Design review of the part built by this model. Coordinates are the model's own, in mm. Face numbers are marked on the shaded views. A direction names the side the tool comes from. Coordinates: 2 decimals unless noted, no trailing zeros. Loops run counter-clockwise (first coordinate to the right, second up) from the corner with the lowest first, then second, coordinate; pieces in that order, holes last. Notation, with made-up numbers: M 19.5,12.25 L 63.5,12.25 A6 cw 63.5,23.25 Z; hole C 50.5,-8.75 d2. An arc over 180 degrees is marked long. Put each result on its own line as item: value. Start each with the question number.
(1) Clearance check with flat-ended pins moving along their axes: pin 1 (1 mm diameter, centred on y = 37, z = 42, fed in from -X); pin 2 (2 mm diameter, centred on y = 20.5, z = 54, fed in from +X); pin 3 (5.5 mm diameter, centred on x = 19.5, y = 46.5, fed in from +Z). State where each tip first meets the part, or that it passes through.
(2) The part is to be moulded in two halves that separate along Z. For the marked faces 4, 5, 6 and 7, say which applies: +Z half, -Z half, draft (parallel to the pull), parting line (faces both ways), or undercut.
(3) Take a section at A-A, the plane y = 21. Give the boundary of the cut face in (x, z), then the cut area to 3 significant figures.
(4) Take a section at C-C, the plane z = 12.5. Give the boundary of the cut face in (x, y).
(5) Take a section at D-D, the plane y = 36.5. Give the boundary of the cut face in (x, z), then the cut area to 3 significant figures.
(6) For probe 1 along Y at (x, z) = (36.5, 46.45); probe 2 along Z at (x, y) = (19.5, 24); probe 3 along X at (y, z) = (5, 47), list the stretches that pass through material, from the lowest coordinate up. Write a range as [from, to].
(7) For the marked faces 1, 2 and 3, list the 3-axis set-ups (+Z, -Z, +X, -X, +Y, -Y) from which the entire face can be reached by the end or side of a thin tool; tool diameter is ignored.
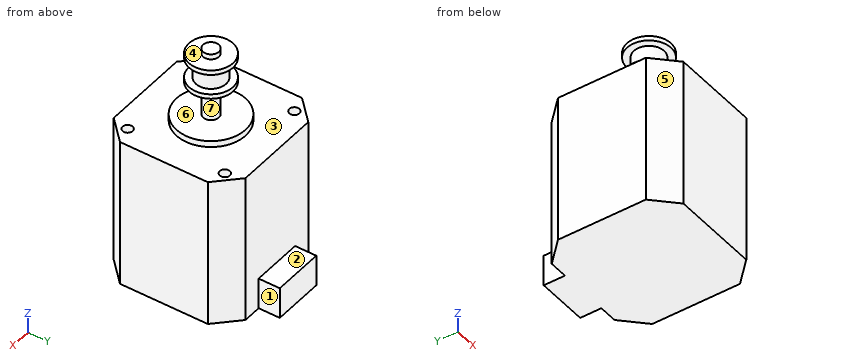
```python
from build123d import *

# Parameters (mm, degrees)
SKETCH1_W           = 42
SKETCH1_H           = 42
BOSS_EXTRUDE1_DEPTH = 47.85
CHAMFER1_SIZE       = 7
SKETCH2_R           = 11
BOSS_EXTRUDE2_DEPTH = 2
SKETCH3_W           = 16.25
SKETCH3_H           = 6.75
BOSS_EXTRUDE3_DEPTH = 10
SKETCH4_R           = 1.6
CUT_EXTRUDE1_DEPTH  = 3


with BuildPart() as part:
    # Sketch1 → Boss-Extrude1 (new body)
    with BuildSketch(Plane.XY):
        with Locations((21, 21)):
            Rectangle(SKETCH1_W, SKETCH1_H)
    extrude(amount=BOSS_EXTRUDE1_DEPTH)

    # Chamfer1
    chamfer1_edges = [part.edges().sort_by_distance(p)[0] for p in [
        (0, 42, 23.925),
        (42, 42, 23.925),
        (42, 0, 23.925),
        (0, 0, 23.925),
    ]]
    chamfer(chamfer1_edges, length=CHAMFER1_SIZE)

    # Sketch2 → Boss-Extrude2 (add)
    with BuildSketch(Plane.XY.offset(47.85)):
        with Locations((21, 21)):
            Circle(SKETCH2_R)
    extrude(amount=BOSS_EXTRUDE2_DEPTH)

    # Sketch3 → Boss-Extrude3 (add)
    with BuildSketch(Plane(origin=(0, 0, 0), x_dir=(-1, 0, 0), z_dir=(0, 0, -1))):
        with Locations((-21, 45.375)):
            Rectangle(SKETCH3_W, SKETCH3_H)
    extrude(amount=-BOSS_EXTRUDE3_DEPTH)

    # Sketch4 → Cut-Extrude1 (cut)
    with BuildSketch(Plane.XY.offset(47.85)):
        with Locations((5.5, 36.5)):
            Circle(SKETCH4_R)
        with Locations((36.5, 36.5)):
            Circle(SKETCH4_R)
        with Locations((36.5, 5.5)):
            Circle(SKETCH4_R)
        with Locations((5.5, 5.5)):
            Circle(SKETCH4_R)
    extrude(amount=-CUT_EXTRUDE1_DEPTH, mode=Mode.SUBTRACT)

    # Sketch5 → Revolve1 (revolve)
    with BuildSketch(Plane(origin=(0, 21, 0), x_dir=(-1, 0, 0), z_dir=(0, -1, 0))):
        Polygon((-18.5, -49.85), (-21, -49.85), (-21, -72.05), (-18.5, -72.05), (-18.5, -70.37), (-14, -70.37), (-14, -68.87), (-16.2, -68.87), (-16.2, -62.32), (-14, -62.32), (-14, -60.82), (-18.5, -60.82), align=None)
    revolve(axis=Axis((21, 21, 49.85), (0, 0, 1)))


solid = part.part
```
Computed values:
1. pin 1: stops at x = 1.5
1. pin 2: stops at x = 23.5
1. pin 3: stops at z = 10
2. face 4: +Z half
2. face 5: draft
2. face 6: undercut
2. face 7: undercut
3. outline: M 0,0 L 42,0 L 42,47.85 L 32,47.85 L 32,49.85 L 23.5,49.85 L 23.5,60.82 L 28,60.82 L 28,62.32 L 25.8,62.32 L 25.8,68.87 L 28,68.87 L 28,70.37 L 23.5,70.37 L 23.5,72.05 L 18.5,72.05 L 18.5,70.37 L 14,70.37 L 14,68.87 L 16.2,68.87 L 16.2,62.32 L 14,62.32 L 14,60.82 L 18.5,60.82 L 18.5,49.85 L 10,49.85 L 10,47.85 L 0,47.85 Z
3. area: 2,220 mm^2
4. outline: M 0,7 L 7,0 L 35,0 L 42,7 L 42,35 L 35,42 L 7,42 L 0,35 Z
5. outline: M 1.5,0 L 40.5,0 L 40.5,47.85 L 38.1,47.85 L 38.1,44.85 L 34.9,44.85 L 34.9,47.85 L 7.1,47.85 L 7.1,44.85 L 3.9,44.85 L 3.9,47.85 L 1.5,47.85 Z
5. area: 1,850 mm^2
6. probe 1: y = [1.5, 3.9], [7.1, 34.9], [38.1, 40.5]
6. probe 2: z = [0, 49.85], [60.82, 70.37]
6. probe 3: x = [2, 3.98], [7.02, 34.98], [38.02, 40]
7. face 1: +Z, -Z, +X, +Y
7. face 2: +Z, +X, -X, +Y
7. face 3: +Z
